Could you check a few things on this drawing? It's one solid part, dimensions in mm from its lowest x, y, z. Give positions to 0.01 mm unless a question says otherwise; leave off trailing zeros. Loops run counter-clockwise (first coordinate to the right, second up) from the corner with the lowest first, then second, coordinate; pieces in that order, holes last. Notation, with made-up numbers: M 32.5,-30 L 87.5,-30 A21 cw 87.5,-26 Z; hole C 41.5,-5 d2. An arc over 180 degrees is marked long. Answer in a Markdown table with one row per item. Add a question column.
1. If we section it at B-B on x = 16: List the corners of the cut face in (y, z) for me.
2. I need wall thicknesses on line 1 along X through (y, z) = (77.5, 90); line 2 along Y through (x, z) = (145.5, 35); line 3 along X through (y, z) = (12, 94). Which ranges of each line are inside material? Lowest first, please. Write a range as from..to.
3. If we section it at A-A on z = 145: List the corners of the cut face in (x, y) for me, then the cut area to 3 significant figures.
4. If we section it at C-C on y = 118: List the corners of the cut face in (x, z) for me, then the cut area to 3 significant figures.
5. I'm going to push flat-ended pins straight in: pin 1 Ø4 at (x, y) = (96.5, 54) entering from -Z; pin 2 Ø4 at (x, z) = (120.5, 114.5) entering from +Y; pin 3 Ø10 at (x, z) = (38, 156) entering from +Y; pin 4 Ø10 at (y, z) = (21, 65) entering from -X. Where does each tip first touch, or does it pass through?
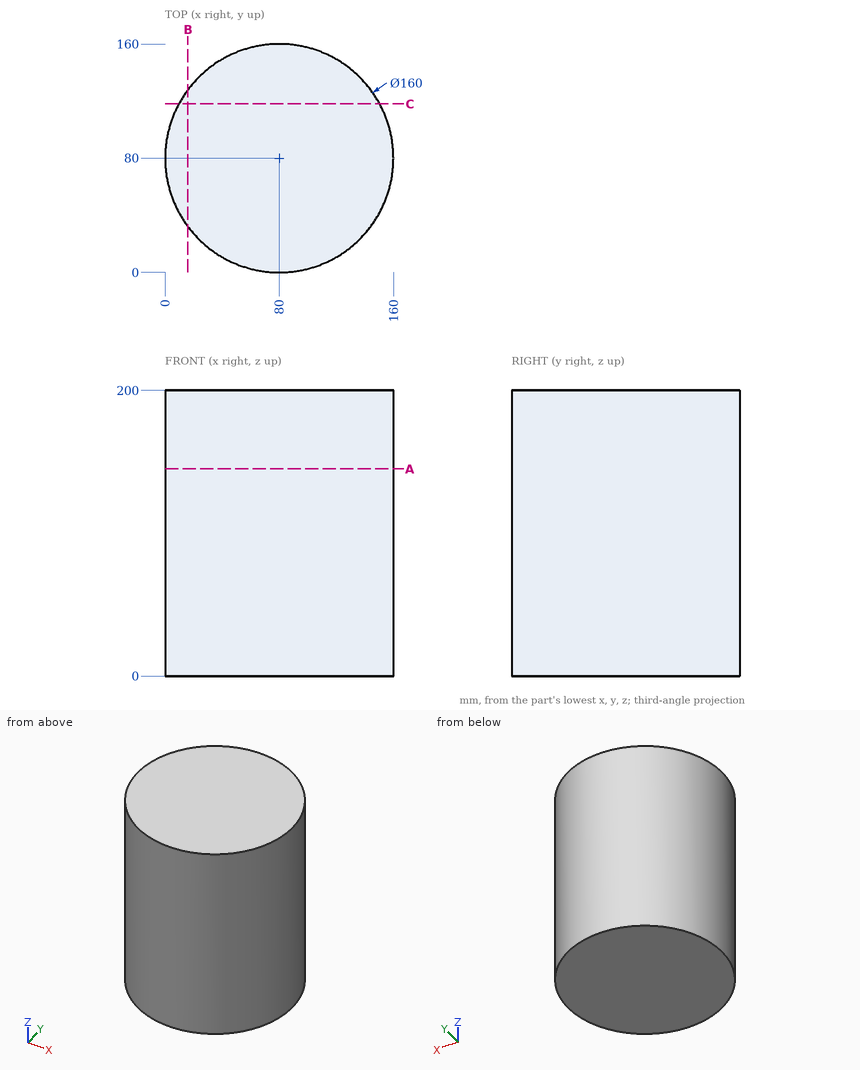
Results:
| question | item | result |
|---|---|---|
| 1 | outline | M 32,0 L 128,0 L 128,200 L 32,200 Z |
| 2 | line 1 | 0.04..159.96 |
| 2 | line 2 | 34.07..125.93 |
| 2 | line 3 | 37.86..122.14 |
| 3 | outline | C 80,80 d160 |
| 3 | area | 20,100 mm2 |
| 4 | outline | M 9.6,0 L 150.4,0 L 150.4,200 L 9.6,200 Z |
| 4 | area | 28,200 mm2 |
| 5 | pin 1 | z = 0 |
| 5 | pin 2 | y = 150.13 |
| 5 | pin 3 | y = 150.93 |
| 5 | pin 4 | x = 20.97 |
